Check sheet for the drawn part. Datum: minimum x, y, z corner. Units: mm. Give positions to 0.01 mm unless a question says otherwise; leave off trailing zeros. Order: outer loops, then holes, each group sorted by start corner. A loop starts at its lowest first (then second) coordinate and runs counter-clockwise, first axis right, second up.
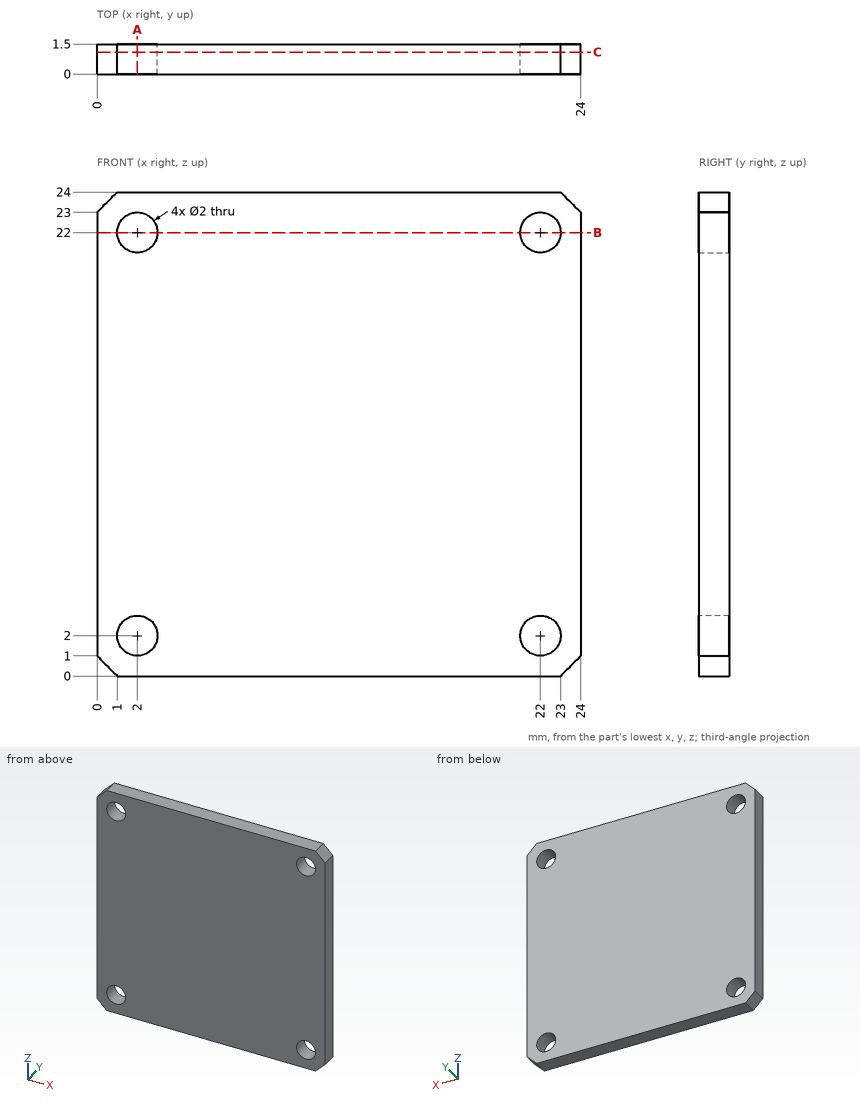
Q1. Sectioned sample at C-C, the plane y = 1.1. Record the cut outline in (x, z).
Q2. Material ranges on line 1 (X direction, y = 0.6, z = 22); line 2 (Z direction, x = 21.75, y = 0.8), recorded low to high.
Q3. Sectioned sample at B-B, the plane z = 22. Record the cut outline in (x, y), plus the area to 3 significant figures.
Q4. Sectioned sample at A-A, the plane x = 2. Record the cut outline in (y, z).
Filled in:
1. outline: (0, 1) - (1, 0) - (23, 0) - (24, 1) - (24, 23) - (23, 24) - (1, 24) - (0, 23) - close; hole circle Ø2 at (2, 2); hole circle Ø2 at (2, 22); hole circle Ø2 at (22, 2); hole circle Ø2 at (22, 22)
2. line 1: x = 0 to 1, 3 to 21, 23 to 24
2. line 2: z = 0 to 1.03, 2.97 to 21.03, 22.97 to 24
3. outline: (0, 0) - (1, 0) - (1, 1.5) - (0, 1.5) - close; (3, 0) - (21, 0) - (21, 1.5) - (3, 1.5) - close; (23, 0) - (24, 0) - (24, 1.5) - (23, 1.5) - close
3. area: 30.0 mm2
4. outline: (0, 0) - (1.5, 0) - (1.5, 1) - (0, 1) - close; (0, 3) - (1.5, 3) - (1.5, 21) - (0, 21) - close; (0, 23) - (1.5, 23) - (1.5, 24) - (0, 24) - close
